Build history of the part. All positions in model axes, mm. A direction names the side the tool comes from. Round coordinates to 2 decimals unless told otherwise and drop trailing zeros. Write each loop counter-clockwise with the first axis right and the second up, starting at its lowest first coordinate (ties: lowest second). Pieces come first, ordered by that corner, then holes. Notation, with made-up numbers: (36.25, 47.25) - (72.25, 47.25) arc R18 cw to (72.25, 60.25) - close; hole circle Ø11 at (16, -19). An arc over 180 degrees is marked (long way). Write each question's results on one line, items separated by ' | '.
Autodesk Inventor part; units mm, degrees
ref_plane "YZ Plane" through (0, 0, 0) normal (1, 0, 0) x (0, 1, 0)
ref_plane "XZ Plane" through (0, 0, 0) normal (0, 1, 0) x (-1, 0, 0)
ref_plane "XY Plane" through (0, 0, 0) normal (0, 0, 1) x (1, 0, 0)
sketch "Sketch1" plane through (0, 0, 0) normal (0, 0, 1) x (1, 0, 0)
  line L0 (-31.225, 0) -> (-22.225, 0)
  line L1 (-22.225, 0) -> (-22.225, 15)
  line L2 (-22.225, 15) -> (-23.225, 15)
  line L3 (-23.225, 15) -> (-23.225, 3)
  line L4 (-23.225, 3) -> (-31.225, 3)
  line L5 (-31.225, 3) -> (-31.225, 0)
  line L6 (0, -3) -> (0, 18)
  point P0 (0, 0)
  dimension "d0" = 3
  dimension "d1" = 1
  dimension "d2" = 15
  dimension "d3" = 22.225
  dimension "d17" = 9
revolve "Revolution1" add sketch "Sketch1" angle 360 about axis through (0, -10, 0) along (0, 1, 0)
sketch "Sketch2" plane through (0, 3, 0) normal (0, 1, 0) x (1, 0, 0)
  point P0 (0, 0)
  point P1 (0, 27)
  dimension "d6" = 27
hole "Hole1" at (0, 3, -27) direction (0, -1, 0) diameter 2.459 end through all
sketch "Sketch3" plane through (0, 15, 0) normal (0, 1, 0) x (1, 0, 0)
  line L0 (-31.225, 0.5) -> (31.225, 0.5)
  line L1 (31.225, 0.5) -> (31.225, -31.225)
  line L2 (31.225, -31.225) -> (-31.225, -31.225)
  line L3 (-31.225, -31.225) -> (-31.225, 0.5)
  circle A0 centre (0, 0) radius 31.225
  circle A1 centre (0, 0) radius 23.225
  point P0 (31.225, 0)
  point P1 (31.221, 0.5)
  point P2 (-31.221, 0.5)
  point P3 (-31.225, 0)
  point P4 (0, -31.225)
  point P5 (23.2196, 0.5)
  point P6 (-23.2196, 0.5)
  dimension "d14" = 0.5
extrude "Extrusion1" cut sketch "Sketch3" against normal blind 15 contours L0 A1 A0 | A0 L2 L3 | L0 A1 | A0 L1 L2 picked at (-27.077, -8.535) picked at (5.7691, -4.8291)
pattern_circular "Circular Pattern1" count 6 over 360 about axis through (0, 7.5, 0) along (0, 1, 0) of "Hole1"
properties part number "LowerClamp" material "Brass, Soft Yellow"
(1) Flat gauge pins, fed straight in: pin 1 Ø8 at (y, z) = (2.5, -27) entering from -X; pin 2 Ø12 at (x, z) = (22.5, -26) entering from -Y; pin 3 Ø3 at (x, z) = (23.38, -13.5) entering from +Y; pin 4 Ø8 at (y, z) = (8, -10.5) entering from +X. Where does each tip first touch, or does it go through?
Worked answers:
pin 1: stops at x = -21.12 | pin 2: stops at y = 0 | pin 3: stops at y = 3 | pin 4: stops at x = 22.3
(2) Tool access for faces 4 (the flat face through (0, 3, -24)), 5 (the flat face through (-25.4, 2.5, -0.5)): list every direction of +Z, -Z, +X, -X, +Y, -Y with a clear straight run to the whole face (end or side of a thin tool).
Worked answers:
face 4: -Z, +Y | face 5: +Z, +X, -X, +Y, -Y
(3) Slice it at C-C, the plane z = -13.5. Write the cut outline in (x, y), and give its area (3 significant figures).
Worked answers:
outline: (-28.16, 0) - (-24.61, 0) - (-24.61, 3) - (-28.16, 3) - close; (-22.15, 0) - (-17.66, 0) - (-17.66, 15) - (-18.9, 15) - (-18.9, 3) - (-22.15, 3) - close; (17.66, 0) - (22.15, 0) - (22.15, 3) - (18.9, 3) - (18.9, 15) - (17.66, 15) - close; (24.61, 0) - (28.16, 0) - (28.16, 3) - (24.61, 3) - close | area: 78.1 mm2
(4) Slice it at D-D, the plane z = -9. Write the cut outline in (x, y).
Worked answers:
outline: (-29.9, 0) - (-20.32, 0) - (-20.32, 15) - (-21.41, 15) - (-21.41, 3) - (-29.9, 3) - close; (20.32, 0) - (29.9, 0) - (29.9, 3) - (21.41, 3) - (21.41, 15) - (20.32, 15) - close
(5) Slice it at B-B, the plane z = -27. Write the cut outline in (x, y), and give its area (3 significant figures).
Worked answers:
outline: (-15.68, 0) - (-1.23, 0) - (-1.23, 3) - (-15.68, 3) - close; (1.23, 0) - (15.68, 0) - (15.68, 3) - (1.23, 3) - close | area: 86.7 mm2
(6) Two-plate mould, pull along X, no slides. Class faces 1 (the cylindrical face through (-0.5, 8.92, -23.22)), 2 (the cylindrical face through (0.471, 1.479, -25.864)), 3 (the flat face through (25, 2.5, -0.5)): released by +X, released by -X, zero draft, split by the parting line, or undercut.
Worked answers:
face 1: split by the parting line | face 2: undercut | face 3: zero draft
(7) Drill centre lines: probe 1 along Z at (x, y) = (0, 0.8) (1 decimal); probe 2 along X at (y, z) = (2.25, -13.5); probe 3 along X at (y, z) = (9.25, -8.5). Where is each one in solid material? Low to high. Write a range as [from, to].
Worked answers:
probe 1: z = [-31.2, -28.2], [-25.8, -22.2] | probe 2: x = [-28.16, -24.61], [-22.15, -17.66], [17.66, 22.15], [24.61, 28.16] | probe 3: x = [-21.61, -20.54], [20.54, 21.61]
(8) Slice it at A-A, the plane x = 0. Write the cut outline in (y, z) (1 decimal), and give its area (3 significant figures).
Worked answers:
outline: (0, -31.2) - (3, -31.2) - (3, -28.2) - (0, -28.2) - close; (0, -25.8) - (3, -25.8) - (3, -23.2) - (15, -23.2) - (15, -22.2) - (0, -22.2) - close | area: 31.6 mm2
